Here's how the part is built. I have some questions about the finished solid (model axes, mm). A direction names the side the tool comes from. Round coordinates to 2 decimals unless told otherwise and drop trailing zeros. Order: outer loops, then holes, each group sorted by start corner. A loop starts at its lowest first (then second) coordinate and runs counter-clockwise, first axis right, second up. Notation, with made-up numbers: (-8, 20) -> (50, 20) arc R23 ccw to (50, 37) -> close; hole circle Ø3 at (37, 13). An arc over 180 degrees is marked (long way). One line per item, written item: value.
```python
from build123d import *

# Parameters (mm, degrees)
F3_W      = 15
F3_H      = 4
F4_DEPTH  = 26.7
F5_W      = 15
F5_H      = 4
F6_DEPTH  = 15
F7_R      = 1.7
F8_DEPTH  = 45.4048897462
F10_DEPTH = 2
F12_DEPTH = 2


with BuildPart() as f2:
    # F2: sweep along a path in F0
    with BuildLine(Plane.XY) as f2_path:
        ThreePointArc((-40, 26.8490467115), (-50, 16.8490467115), (-40, 6.8490467115))
        Line((-40, 6.8490467115), (40, 6.8490467115))
        ThreePointArc((40, 6.8490467115), (50, 16.8490467115), (40, 26.8490467115))
        Line((40, 26.8490467115), (-40, 26.8490467115))
    # F1 (on Right) → F2 (sweep)
    with BuildSketch(Plane.YZ):
        with BuildLine():
            Line((4.4971018384, 2), (4.4971018384, -2))
            Line((4.4971018384, -2), (9.4971018384, -2))
            Line((9.4971018384, -2), (9.4971018384, 0))
            ThreePointArc((9.4971018384, 0), (9.2955306442, 1.013366825), (8.7215044486, 1.8724577372))
            Line((8.7215044486, 1.8724577372), (8.5939621858, 2))
            Line((8.5939621858, 2), (4.4971018384, 2))
        make_face()
    sweep(path=f2_path.line)

    # F3 (on face) → F4 (join)
    with BuildSketch(Plane.XZ.offset(-4.4971018384)):
        with Locations((-17.5, 0)):
            Rectangle(F3_W, F3_H)
        with Locations((17.5, 0)):
            Rectangle(F3_W, F3_H)
    extrude(amount=F4_DEPTH)

    # F5 (on face) → F6 (join)
    with BuildSketch(Plane(origin=(0, 0, -2), x_dir=(1, 0, 0), z_dir=(0, 0, -1))):
        with Locations((-17.5, 14.2028981616)):
            Rectangle(F5_W, F5_H)
        with Locations((-17.5, 3.5028981616)):
            Rectangle(F5_W, F5_H)
        with Locations((17.5, 14.2028981616)):
            Rectangle(F5_W, F5_H)
        with Locations((17.5, 3.5028981616)):
            Rectangle(F5_W, F5_H)
    extrude(amount=F6_DEPTH)

    # F7 (on face) → F8 (cut, through all)
    with BuildSketch(Plane.XZ.offset(16.2028981616)):
        with Locations((-17.5, -9.5)):
            Circle(F7_R)
        with Locations((17.5, -9.5)):
            Circle(F7_R)
    extrude(amount=-F8_DEPTH, mode=Mode.SUBTRACT)

    # F9 (on face) → F10 (join)
    with BuildSketch(Plane(origin=(-25, 0, 0), x_dir=(0, -1, 0), z_dir=(-1, 0, 0))):
        Polygon((1.5028981616, -12.3923048454), (1.5028981616, -2), (-4.4971018384, -2), align=None)
        Polygon((22.2028981616, -2), (16.2028981616, -2), (16.2028981616, -12.3923048454), align=None)
    extrude(amount=-F10_DEPTH)

    # F11 (on face) → F12 (join)
    with BuildSketch(Plane.YZ.offset(25)):
        Polygon((-16.2028981616, -12.3923048454), (-16.2028981616, -2), (-22.2028981616, -2), align=None)
        Polygon((-1.5028981616, -12.3923048454), (4.4971018384, -2), (-1.5028981616, -2), align=None)
    extrude(amount=-F12_DEPTH)


solid = f2.part
```
Q1. I want a section at A-A on y = -6.5. Write out the boundary of the cut face in (x, z).
Answers:
outline: (-25, -2) -> (-10, -2) -> (-10, 2) -> (-25, 2) -> close; (10, -2) -> (25, -2) -> (25, 2) -> (10, 2) -> close
Q2. I want a section at D-D on y = 1.5. Write out the boundary of the cut face in (x, z), then the cut area to 3 significant figures.
Answers:
outline: (-25, -7.19) -> (-23, -7.19) -> (-23, -2) -> (-10, -2) -> (-10, 2) -> (-25, 2) -> close; (10, -2) -> (23, -2) -> (23, -7.19) -> (25, -7.19) -> (25, 2) -> (10, 2) -> close
area: 141 mm2
Q3. I want a section at C-C on z = -4.5. Write out the boundary of the cut face in (x, y).
Answers:
outline: (-25, -20.76) -> (-23, -20.76) -> (-23, -16.2) -> (-10, -16.2) -> (-10, -12.2) -> (-25, -12.2) -> close; (-25, -5.5) -> (-10, -5.5) -> (-10, -1.5) -> (-23, -1.5) -> (-23, 3.05) -> (-25, 3.05) -> close; (10, -16.2) -> (23, -16.2) -> (23, -20.76) -> (25, -20.76) -> (25, -12.2) -> (10, -12.2) -> close; (10, -5.5) -> (25, -5.5) -> (25, 3.05) -> (23, 3.05) -> (23, -1.5) -> (10, -1.5) -> close
Q4. For P1, Ø4.5, axis at x = -14, z = -8.5, coming from the -Y side; P2, Ø1.5, axis at x = -10, z = -2.5, coming from the +Y side; P3, Ø9, axis at x = -13.5, y = 13.5, coming from the -Z side; P4, Ø1.2, axis at x = 2.5, z = 1, coming from the -Y side, each with a flat end and sliding along its axis, tell me the tip position at first contact or that it passes through.
Answers:
P1: y = -16.2
P2: y = 29.2
P3: z = -2
P4: y = 4.5
Q5. I want a section at B-B on x = 12. Write out the boundary of the cut face in (y, z).
Answers:
outline: (-22.2, -2) -> (-16.2, -2) -> (-16.2, -17) -> (-12.2, -17) -> (-12.2, -2) -> (-5.5, -2) -> (-5.5, -17) -> (-1.5, -17) -> (-1.5, -2) -> (9.5, -2) -> (9.5, 0) arc R2.65 ccw to (8.72, 1.87) -> (8.59, 2) -> (-22.2, 2) -> close; (24.2, -2) -> (29.2, -2) -> (29.2, 2) -> (25.1, 2) -> (24.98, 1.87) arc R2.65 ccw to (24.2, 0) -> close
Q6. Which directions (+Z, -Z, +X, -X, +Y, -Y) give clear straight access to the entire face, cutting with the end or side of a thin tool? Please do faces 1 (the face through (18, -9, -2)), 2 (the face through (-0.56, 24.397, 1)), 3 (the face through (25, -9, -1)).
Answers:
face 1: -Z, +X, -X
face 2: +Z
face 3: +Z, -Z, +X, -Y
Q7. If we mould it in two halves opening along X, with no side actions, what happens to faces 4 (the face through (33, 4.497, 0)), 5 (the face through (-23, -18, -6)), 6 (the face through (-52.35, 17.12, -0.03))? For each: pulls with the +X half, pulls with the -X half, needs draft (parallel to the pull), parting line crosses it, or undercut.
Answers:
face 4: needs draft
face 5: undercut
face 6: pulls with the -X half
Q8. I need wall thicknesses on line 1 along X through (y, z) = (-5, -9.25); line 2 along X through (y, z) = (-14.5, -7.25); line 3 along Y through (x, z) = (19.5, -10.5). Which ranges of each line are inside material? Lowest first, please.
Answers:
line 1: -25 to -19.18, -15.82 to -10, 10 to 15.82, 19.18 to 25
line 2: -25 to -10, 10 to 25
line 3: -16.2 to -12.2, -5.5 to -1.5
